```python
from build123d import *

# Parameters (mm, degrees)
F0_R     = 10.25
F0_R_2   = 3.925
F0_R_3   = 3.15
F1_DEPTH = 5
F2_DEPTH = 4.6
F3_R     = 1.5
F4_DEPTH = 12.5
F5_COUNT = 10
F5_ANGLE = 324


with BuildPart() as f1:
    # F0 (on Front) → F1 (new body, symmetric)
    with BuildSketch(Plane.XZ):
        Circle(F0_R)
        Circle(F0_R_2, mode=Mode.SUBTRACT)
        Circle(F0_R_2)
        Circle(F0_R_3, mode=Mode.SUBTRACT)
    extrude(amount=F1_DEPTH, both=True)

    # F0 (on Front) → F2 (cut, symmetric)
    with BuildSketch(Plane.XZ):
        Circle(F0_R)
        Circle(F0_R_2, mode=Mode.SUBTRACT)
    extrude(amount=F2_DEPTH, both=True, mode=Mode.SUBTRACT)


with BuildPart() as f4:
    # F3 (on face) → F4 (new body, symmetric)
    with BuildSketch(Plane.XZ.offset(5)):
        with Locations((0, 7.75)):
            Circle(F3_R)
    extrude(amount=F4_DEPTH, both=True)


with BuildPart() as f5_1:
    # F5: instance of F4
    add(f4.part.rotate(Axis((0, -5, 0), (0, -1, 0)), 1 * F5_ANGLE / (F5_COUNT - 1)))


with BuildPart() as f5_2:
    # F5: instance of F4
    add(f4.part.rotate(Axis((0, -5, 0), (0, -1, 0)), 2 * F5_ANGLE / (F5_COUNT - 1)))


with BuildPart() as f5_3:
    # F5: instance of F4
    add(f4.part.rotate(Axis((0, -5, 0), (0, -1, 0)), 3 * F5_ANGLE / (F5_COUNT - 1)))


with BuildPart() as f5_4:
    # F5: instance of F4
    add(f4.part.rotate(Axis((0, -5, 0), (0, -1, 0)), 4 * F5_ANGLE / (F5_COUNT - 1)))


with BuildPart() as f5_5:
    # F5: instance of F4
    add(f4.part.rotate(Axis((0, -5, 0), (0, -1, 0)), 5 * F5_ANGLE / (F5_COUNT - 1)))


with BuildPart() as f5_6:
    # F5: instance of F4
    add(f4.part.rotate(Axis((0, -5, 0), (0, -1, 0)), 6 * F5_ANGLE / (F5_COUNT - 1)))


with BuildPart() as f5_7:
    # F5: instance of F4
    add(f4.part.rotate(Axis((0, -5, 0), (0, -1, 0)), 7 * F5_ANGLE / (F5_COUNT - 1)))


with BuildPart() as f5_8:
    # F5: instance of F4
    add(f4.part.rotate(Axis((0, -5, 0), (0, -1, 0)), 8 * F5_ANGLE / (F5_COUNT - 1)))


with BuildPart() as f5_9:
    # F5: instance of F4
    add(f4.part.rotate(Axis((0, -5, 0), (0, -1, 0)), 9 * F5_ANGLE / (F5_COUNT - 1)))


with BuildPart() as f1_1:
    add(f1.part)

    # F6: cut F4, F5_1, F5_2, F5_3, F5_4, F5_5, F5_6, F5_7, F5_8, F5_9
    add(f4.part, mode=Mode.SUBTRACT)
    add(f5_1.part, mode=Mode.SUBTRACT)
    add(f5_2.part, mode=Mode.SUBTRACT)
    add(f5_3.part, mode=Mode.SUBTRACT)
    add(f5_4.part, mode=Mode.SUBTRACT)
    add(f5_5.part, mode=Mode.SUBTRACT)
    add(f5_6.part, mode=Mode.SUBTRACT)
    add(f5_7.part, mode=Mode.SUBTRACT)
    add(f5_8.part, mode=Mode.SUBTRACT)
    add(f5_9.part, mode=Mode.SUBTRACT)


solid = f1_1.part
```
Model file for the job. Use its own axes, mm. Give positions to 0.01 mm unless a question says otherwise; leave off trailing zeros. Order: outer loops, then holes, each group sorted by start corner. A loop starts at its lowest first (then second) coordinate and runs counter-clockwise, first axis right, second up.
1) Pin check, flat tips, straight feed: pin 1 (4 mm diameter, centred on y = -2, z = -6.5, fed in from -X); pin 2 (4 mm diameter, centred on x = 4.56, z = -6.27, fed in from +Y); pin 3 (1 mm diameter, centred on y = 1.5, z = -1, fed in from +X); pin 4 (4 mm diameter, centred on y = -4, z = 7.5, fed in from +X). Stop position of each tip, or through.
2) Mould opens along Z. For faces 1 (the cylindrical face through (-2.222, 4.797, -10.006)), 2 (the flat face through (-2.4, 5, 2.4)), 3 (the cylindrical face through (-3.7, -4.8, 7.5)) say: +Z half, -Z half, draft (parallel to the pull), parting line (faces both ways), or undercut.
3) Saw through at D-D, the plane y = 0.25. Write the cut outline in (x, z) (3 decimals).
4) Wall check: probe 1 along Z at (x, y) = (0, 4.9); probe 2 along Y at (x, z) = (1.75, -9); probe 3 along X at (y, z) = (-3, -2.25). Give the ranges that are in metal, low to high.
5) Saw through at A-A, the plane z = -1.75. Count the separate pieces of the cut face and the enclosed holes in it, then the cut area to 3 significant figures.
Computed:
1. pin 1: passes through
1. pin 2: stops at y = 5
1. pin 3: stops at x = 3.89
1. pin 4: stops at x = 8.59
2. face 1: parting line
2. face 2: draft
2. face 3: undercut
3. outline: circle Ø7.85 at (0, 0); hole circle Ø6.3 at (0, 0)
4. probe 1: z = -10.25 to -9.25, -6.25 to -3.15, 3.15 to 6.25, 9.25 to 10.25
4. probe 2: y = -5 to -4.6, 4.6 to 5
4. probe 3: x = -3.22 to -2.2, 2.2 to 3.22
5. separate pieces: 6
5. enclosed holes: 0
5. area: 24.1 mm2
